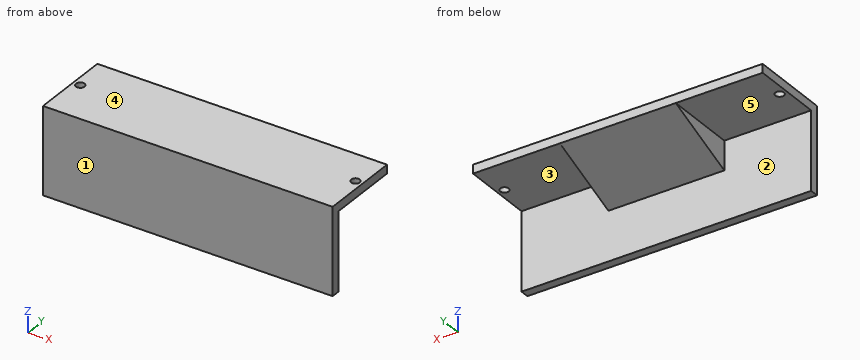
```python
from build123d import *

# Parameters (mm, degrees)
SKETCH1_W           = 100
SKETCH1_H           = 25
SKETCH1_R           = 1.5
BOSS_EXTRUDE1_DEPTH = 3
SKETCH2_W           = 100
SKETCH2_H           = 30
BOSS_EXTRUDE2_DEPTH = 3
RIB1_REACH          = 60.9
SKETCH3_WALL_W      = 146.72650315
SKETCH3_WALL_H      = 40


with BuildPart() as part:
    # Sketch1 → Boss-Extrude1 (new body)
    with BuildSketch(Plane.XY):
        Rectangle(SKETCH1_W, SKETCH1_H)
        with Locations((-47.5, 0)):
            Circle(SKETCH1_R, mode=Mode.SUBTRACT)
        with Locations((47.5, 0)):
            Circle(SKETCH1_R, mode=Mode.SUBTRACT)
    extrude(amount=BOSS_EXTRUDE1_DEPTH)

    # Sketch2 → Boss-Extrude2 (add)
    with BuildSketch(Plane.XZ.offset(12.5)):
        with Locations((0, -12)):
            Rectangle(SKETCH2_W, SKETCH2_H)
    extrude(amount=BOSS_EXTRUDE2_DEPTH)

    # Sketch3 wall → Rib1 (add, up to next)
    with BuildSketch(Plane(origin=(0, 0, -5), x_dir=(0, -0.928476690885, -0.371390676354), z_dir=(0, 0.371390676354, -0.928476690885)), mode=Mode.PRIVATE) as rib1_sk1:
        Rectangle(SKETCH3_WALL_W, SKETCH3_WALL_H)
    rib1_tool1 = extrude(rib1_sk1.sketch, amount=-RIB1_REACH, mode=Mode.PRIVATE) - part.part
    add(rib1_tool1.solids().sort_by_distance((0, 0, -5))[0])


solid = part.part
```
Geometry: final body of the model. Coordinates: model frame, mm. Face numbers are marked on the shaded views. A direction names the side the tool comes from. Round coordinates to 2 decimals unless told otherwise and drop trailing zeros. Loops run counter-clockwise (first coordinate to the right, second up) from the corner with the lowest first, then second, coordinate; pieces in that order, holes last.
Item 1: Section B-B, the plane x = 47.5. Output: boundary loops of the cut face in (y, z).
Checked values:
outline: (-15.5, -27) - (-12.5, -27) - (-12.5, 0) - (-1.5, 0) - (-1.5, 3) - (-15.5, 3) - close; (1.5, 0) - (12.5, 0) - (12.5, 3) - (1.5, 3) - close
Item 2: Contact query for flat-ended pins moving along their axis: P1, Ø10, axis at x = 25.5, y = 3.5, coming from the -Z side; P2, Ø12, axis at x = -26.5, z = -18, coming from the +Y side. Output: stop coordinate, or through.
Checked values:
P1: stops at z = 0
P2: stops at y = -12.5
Item 3: Section D-D, the plane x = -4. Output: boundary loops of the cut face in (y, z).
Checked values:
outline: (-15.5, -27) - (-12.5, -27) - (-12.5, -10) - (12.5, 0) - (12.5, 3) - (-15.5, 3) - close
Item 4: Section A-A, the plane y = 0. Output: boundary loops of the cut face in (x, z), plus the area to 3 significant figures.
Checked values:
outline: (-50, 0) - (-49, 0) - (-49, 3) - (-50, 3) - close; (-46, 0) - (-20, 0) - (-20, -5) - (20, -5) - (20, 0) - (46, 0) - (46, 3) - (-46, 3) - close; (49, 0) - (50, 0) - (50, 3) - (49, 3) - close
area: 482 mm2
Item 5: Section C-C, the plane y = -11.5. Output: boundary loops of the cut face in (x, z), plus the area to 3 significant figures.
Checked values:
outline: (-50, 0) - (-20, 0) - (-20, -9.6) - (20, -9.6) - (20, 0) - (50, 0) - (50, 3) - (-50, 3) - close
area: 684 mm2
Item 6: Line query: L1, parallel to Y at x = -47.5, z = 1.95; L2, parallel to Y at x = 36, z = -22.75; L3, parallel to Z at x = 36, y = 2.5. Output: solid intervals per line, ascending.
Checked values:
L1: y = -15.5 to -1.5, 1.5 to 12.5
L2: y = -15.5 to -12.5
L3: z = 0 to 3
Item 7: Reachability of the marked faces 1, 2, 3, 4 and 5 from +Z, -Z, +X, -X, +Y, -Y: full face, straight path, thin tool, end or side. Return the list, or none.
Checked values:
face 1: +Z, -Z, +X, -X, -Y
face 2: -Z, +Y
face 3: -Z, +X, +Y
face 4: +Z, +X, -X, +Y, -Y
face 5: -Z, -X, +Y
